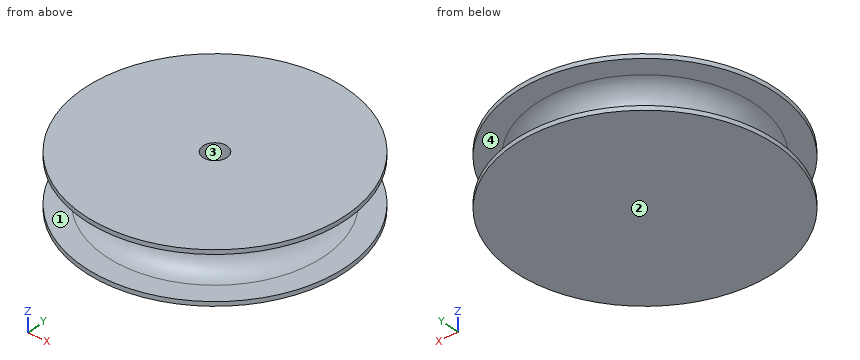
from build123d import *

# Parameters (mm, degrees)
F0_R      = 50.8
F1_DEPTH  = 30.48
F0_R_2    = 76.2
F2_DEPTH  = 2.54
F3_R      = 76.2
F4_DEPTH  = 2.54
F5_R      = 12.69999
F6_R      = 1.27
F7_DEPTH  = 254
F8_DEPTH  = 254
F9_R      = 6.9999987
F10_DEPTH = 27.94


# Not quite as in the source:
# - a fillet or chamfer is up to 0.001 mm smaller than in the source, because OpenCascade refuses the exact size


with BuildPart() as f1:
    # F0 (on Top) → F1 (new body)
    with BuildSketch(Plane.XY):
        Circle(F0_R)
    extrude(amount=F1_DEPTH)

    # F0 (on Top) → F2 (join)
    with BuildSketch(Plane.XY):
        Circle(F0_R_2)
        Circle(F0_R, mode=Mode.SUBTRACT)
    extrude(amount=F2_DEPTH)

    # F3 (on face) → F4 (join)
    with BuildSketch(Plane.XY.offset(30.48)):
        Circle(F3_R)
    extrude(amount=-F4_DEPTH)

    # F5 (radius 12.7 in the source; OpenCascade refuses exactly that, so slightly less here)
    f5_edges = [f1.edges().sort_by_distance(p)[0] for p in [
        (50.8, 0, 15.24),
        (-50.8, 0, 27.94),
        (-50.8, 0, 2.54),
    ]]
    fillet(f5_edges, radius=F5_R)

    # F6 (on Right) → F7 (cut)
    with BuildSketch(Plane.YZ):
        with Locations((0, 15.24)):
            Circle(F6_R)
    extrude(amount=-F7_DEPTH, mode=Mode.SUBTRACT)

    # F6 (on Right) → F8 (cut)
    with BuildSketch(Plane.YZ):
        with Locations((0, 15.24)):
            Circle(F6_R)
    extrude(amount=F8_DEPTH, mode=Mode.SUBTRACT)

    # F9 (on face) → F10 (cut)
    with BuildSketch(Plane.XY.offset(30.48)):
        Circle(F9_R)
    extrude(amount=-F10_DEPTH, mode=Mode.SUBTRACT)


solid = f1.part
Check sheet for the modelled part. Datum: model origin and axes. Units: mm. Face numbers are marked on the shaded views. Give positions to 0.01 mm unless a question says otherwise; leave off trailing zeros. Write each loop counter-clockwise with the first axis right and the second up, starting at its lowest first coordinate (ties: lowest second). Pieces come first, ordered by that corner, then holes. Notation, with made-up numbers: M -34,3 L 8,3 A34 cw 8,36 Z; hole C 67,69 d5. An arc over 180 degrees is marked long. Use one line per item in the form item = value.
(1) Depth check by flat-ended pin: P1, Ø10, axis at y = 41.5, z = 14.5, coming from the -X side; P2, Ø1, axis at y = -8.5, z = 8, coming from the +X side; P3, Ø1, axis at y = -54.5, z = 21.5, coming from the +X side; P4, Ø5, axis at y = -16.5, z = 10, coming from the -X side. Enter the tip coordinate at first touch or a pass-through.
Answer block:
P1 = -35.4
P2 = 52.76
P3 = through
P4 = -50.97
(2) Draft check along Z on the marked faces 1, 2, 3 and 4. Enter one of: pulls with the +Z half, pulls with the -Z half, needs draft (parallel to the pull), parting line crosses it, or undercut.
Answer block:
face_1 = undercut
face_2 = pulls with the -Z half
face_3 = needs draft
face_4 = undercut
(3) Material ranges on line 1 along Z through (x, y) = (18, 0); line 2 along Z through (x, y) = (64, -18.5); line 3 along Z through (x, y) = (0.5, 2.5), recorded low to high.
Answer block:
line_1 = 0 to 13.97, 16.51 to 30.48
line_2 = 0 to 2.54, 27.94 to 30.48
line_3 = 0 to 2.54
(4) Section check B-B on z = 23. Record the boundary of the cut face in (x, y).
Answer block:
outline = C 0,0 d106.89; hole C 0,0 d14
